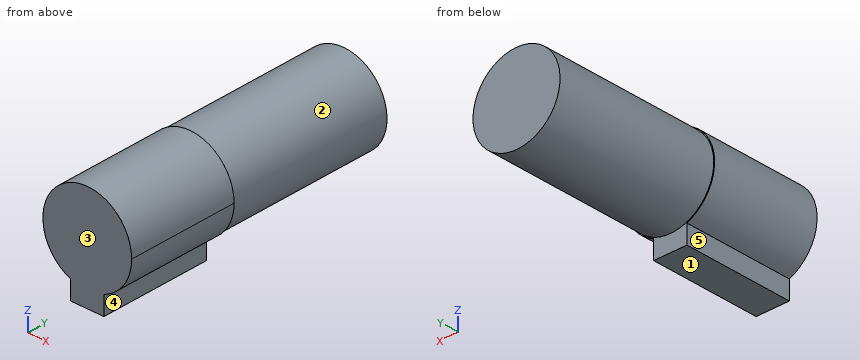
from build123d import *

# Parameters (mm, degrees)
EXTRUDE_1_DEPTH = 10
SKETCH_3_R      = 3.925
EXTRUDE_2_DEPTH = 15


with BuildPart() as part:
    # 草图1 → 凸台-拉伸1 (new body)
    with BuildSketch(Plane(origin=(0, 0, 0), x_dir=(1, 0, 0), z_dir=(0, 1, 0))):
        with BuildLine():
            ThreePointArc((1.5, 3.708099244), (0, 4), (-1.5, 3.708099244))
            Line((-1.5, 3.708099244), (-1.5, 0))
            Line((-1.5, 0), (1.5, 0))
            Line((1.5, 0), (1.5, 3.708099244))
        make_face()
        with BuildLine():
            Line((-1.5, 0), (-1.5, 3.708099244))
            ThreePointArc((-1.5, 3.708099244), (-2.236067977, -3.31662479), (4, 0))
            ThreePointArc((4, 0), (3.31662479, 2.236067977), (1.5, 3.708099244))
            Line((1.5, 3.708099244), (1.5, 0))
            Line((1.5, 0), (-1.5, 0))
        make_face()
        with BuildLine():
            ThreePointArc((1.5, 3.708099244), (0, 4), (-1.5, 3.708099244))
            Line((-1.5, 3.708099244), (-1.5, 0))
            Line((-1.5, 0), (1.5, 0))
            Line((1.5, 0), (1.5, 3.708099244))
        make_face()
        with BuildLine():
            Line((-1.5, 0), (-1.5, 3.708099244))
            ThreePointArc((-1.5, 3.708099244), (-2.236067977, -3.31662479), (4, 0))
            ThreePointArc((4, 0), (3.31662479, 2.236067977), (1.5, 3.708099244))
            Line((1.5, 3.708099244), (1.5, 0))
            Line((1.5, 0), (-1.5, 0))
        make_face()
        with BuildLine():
            Line((1.5, 5.4), (-1.5, 5.4))
            Line((-1.5, 5.4), (-1.5, 3.708099244))
            ThreePointArc((-1.5, 3.708099244), (0, 4), (1.5, 3.708099244))
            Line((1.5, 3.708099244), (1.5, 5.4))
        make_face()
    extrude(amount=EXTRUDE_1_DEPTH)

    # 草图3 → 凸台-拉伸2 (add)
    with BuildSketch(Plane(origin=(0, 10, 0), x_dir=(1, 0, 0), z_dir=(0, 1, 0))):
        with Locations(Location((0, 0, 0), (0, 0, 270))):
            Circle(SKETCH_3_R)
    extrude(amount=EXTRUDE_2_DEPTH)


solid = part.part
Source: CAD feature listing. Evaluate the final solid. Frame: model axes, mm. Face numbers are marked on the shaded views. A direction names the side the tool comes from. Give positions to 0.01 mm unless a question says otherwise; leave off trailing zeros. Write each loop counter-clockwise with the first axis right and the second up, starting at its lowest first coordinate (ties: lowest second). Pieces come first, ordered by that corner, then holes. Notation, with made-up numbers: M 87,0 L 92,0 A8 ccw 92,10 Z; hole C 17.5,40.5 d5. An arc over 180 degrees is marked long. Return JSON: item names as keys, results as strings. Group by question number.
1) Pin query (flat end, axial travel): P1, Ø1.4, axis at y = 7.5, z = -4.5, coming from the +X side; P2, Ø2, axis at y = 20.5, z = -1.5, coming from the +X side; P3, Ø5, axis at y = 10.5, z = -4.5, coming from the +X side; P4, Ø4, axis at x = -3, y = 3, coming from the -Z side. Return the tip coordinate at first contact, or that it passes through.
2) Cut plane B-B, the plane x = 0. Output: boundary loops of the cut face in (y, z) (3 decimals), plus the area to 3 significant figures.
3) Material intervals for line 1 along Y through (x, z) = (0.25, -5); line 2 along Z through (x, y) = (1.5, 19.25); line 3 along X through (y, z) = (23, 3.25), sorted ascending. Write a range as [from, to].
4) Cut plane A-A, the plane z = 2.75. Output: boundary loops of the cut face in (x, y).
5) Cut plane D-D, the plane y = 20.25. Output: boundary loops of the cut face in (x, z) (3 decimals), plus the area to 3 significant figures.
6) Cut plane C-C, the plane y = 6. Output: boundary loops of the cut face in (x, z).
7) Set-up query: the marked faces 1, 2, 3, 4 and 5. Return all of +Z, -Z, +X, -X, +Y, -Y with unobstructed straight access to the full face (end or side cutting, diameter ignored); none if empty.
Recorded:
{
 "1": {"P1": "stops at x = 1.5", "P2": "stops at x = 3.89", "P3": "stops at x = 3.43", "P4": "stops at z = -5.4"},
 "2": {"outline": "M 0,-5.4 L 10,-5.4 L 10,-3.925 L 25,-3.925 L 25,3.925 L 10,3.925 L 10,4 L 0,4 Z", "area": "212 mm²"},
 "3": {"line 1": "y = [0, 10]", "line 2": "z = [-3.63, 3.63]", "line 3": "x = [-2.2, 2.2]"},
 "4": {"outline": "M -2.9,0 L 2.9,0 L 2.9,10 L 2.8,10 L 2.8,25 L -2.8,25 L -2.8,10 L -2.9,10 Z"},
 "5": {"outline": "C 0,0 d7.85", "area": "48.4 mm²"},
 "6": {"outline": "M -1.5,-5.4 L 1.5,-5.4 L 1.5,-3.71 A4 ccw long -1.5,-3.71 Z"},
 "7": {"face 1": "-Z, +X, -X, +Y, -Y", "face 2": "+Y", "face 3": "+Z, -Z, +X, -X, -Y", "face 4": "-Z, +X, +Y, -Y", "face 5": "-Z, -X, +Y, -Y"}
}
